Autodesk Inventor part; units mm, degrees
ref_plane "YZ Plane" through (0, 0, 0) normal (1, 0, 0) x (0, 1, 0)
ref_plane "XZ Plane" through (0, 0, 0) normal (0, 1, 0) x (-1, 0, 0)
ref_plane "XY Plane" through (0, 0, 0) normal (0, 0, 1) x (1, 0, 0)
sketch "스케치1" plane through (0, 0, 0) normal (0, 0, 1) x (1, 0, 0)
  circle A0 centre (0, 0) radius 1.25
  circle A1 centre (5.5, 0) radius 1.25
  line L0 (0, 1.25) -> (5.5, 1.25)
  line L1 (0, -1.25) -> (5.5, -1.25)
  dimension "d0" = 5.5
  dimension "d1" = 2.5
extrude "돌출1" add sketch "스케치1" along normal blind 1
extrude "돌출2" add sketch "스케치1" against normal blind 2 contours A0 | A1
properties part number "ModuleConnector_Axis_Connector_3D 인쇄"
Could you check a few things on this model? Use its own coordinates, in mm. Coordinates: 2 decimals unless noted, no trailing zeros. Order: outer loops, then holes, each group sorted by start corner. A loop starts at its lowest first (then second) coordinate and runs counter-clockwise, first axis right, second up. Notation, with made-up numbers: (-29, -3.75) - (12, -3.75) arc R14 cw to (12, 7.25) - close; hole circle Ø11 at (45.25, -31.75). An arc over 180 degrees is marked (long way). Answer in a Markdown table with one row per item. Add a question column.
(1) Will these pins go through, and if not, where does the flat tip stop? pin 1 (1.2 mm diameter, centred on x = 2.5, y = 0, fed in from -Z); pin 2 (1.5 mm diameter, centred on x = 4.5, z = -1.5, fed in from +Y).
(2) If we section it at C-C, the plane z = 0.5: Please give me the cut outline in (x, y), then the cut area to 3 significant figures.
(3) I need wall thicknesses on L1, parallel to Z at x = 3.25, y = -0.35; L2, parallel to X at y = 0.75, z = -1.25; L3, parallel to X at y = -0.4, z = -0.8. Which ranges of each line are inside material? Lowest first, please.
(4) If we section it at D-D, the plane x = 1.75: Please give me the cut outline in (y, z), then the cut area to 3 significant figures.
(5) If we mould it in two halves opening along X, with no side actions, what happens to faces 1 (the face through (6.66, -0.47, -0.52)), 2 (the face through (0, 0, -2)), 3 (the face through (-1.25, -0.05, -0.85))? For each: released by +X, released by -X, zero draft, split by the parting line, or undercut.
(6) If we section it at B-B, the plane y = 0: Please give me the cut outline in (x, z), then the cut area to 3 significant figures.
(7) If we section it at A-A, the plane z = -0.6: Please give me the cut outline in (x, y).
Results are:
| question | item | result |
|---|---|---|
| 1 | pin 1 | stops at z = 0 |
| 1 | pin 2 | stops at y = 1.22 |
| 2 | outline | (0, -1.25) - (5.5, -1.25) arc R1.25 ccw to (5.5, 1.25) - (0, 1.25) arc R1.25 ccw to start |
| 2 | area | 18.7 mm2 |
| 3 | L1 | z = 0 to 1 |
| 3 | L2 | x = -1 to 1, 4.5 to 6.5 |
| 3 | L3 | x = -1.18 to 1.18, 4.32 to 6.68 |
| 4 | outline | (-1.25, 0) - (1.25, 0) - (1.25, 1) - (-1.25, 1) - close |
| 4 | area | 2.50 mm2 |
| 5 | face 1 | undercut |
| 5 | face 2 | zero draft |
| 5 | face 3 | undercut |
| 6 | outline | (-1.25, -2) - (1.25, -2) - (1.25, 0) - (4.25, 0) - (4.25, -2) - (6.75, -2) - (6.75, 1) - (-1.25, 1) - close |
| 6 | area | 18.0 mm2 |
| 7 | outline | circle Ø2.5 at (0, 0); circle Ø2.5 at (5.5, 0) |
